Could you check a few things on this model? Use its own coordinates, in mm. Face numbers are marked on the shaded views. A direction names the side the tool comes from. Give positions to 0.01 mm unless a question says otherwise; leave off trailing zeros. Loops run counter-clockwise (first coordinate to the right, second up) from the corner with the lowest first, then second, coordinate; pieces in that order, holes last. Notation, with made-up numbers: (1.25, 71.5) - (33.25, 71.5) arc R16 ccw to (33.25, 81.5) - close; hole circle Ø10 at (24.5, -26.5). An arc over 180 degrees is marked (long way). Write each question's results on one line, items separated by ' | '. Start each with the question number.
(1) I need wall thicknesses on line 1 (X direction, y = -15, z = 22.25); line 2 (Y direction, x = 15, z = 22.2); line 3 (Y direction, x = -10, z = 13). Which ranges of each line are inside material? Lowest first, please.
(2) For pin 1 (1.8 mm diameter, centred on x = 15, y = -15, fed in from +Z); pin 2 (5 mm diameter, centred on x = -20, y = -15, fed in from +Z); pin 3 (10 mm diameter, centred on y = 21.5, z = 11.5, fed in from -X), each with a flat end and sliding along its axis, tell me the tip position at first contact or that it passes through.
(3) Suppose I cut it at C-C (z = 18.75). Please give me the cut outline in (x, y), and give its area (3 significant figures).
(4) Suppose I cut it at A-A (y = -15). Please give me the cut outline in (x, z).
(5) Suppose I cut it at B-B (x = 15). Please give me the cut outline in (y, z).
(6) Suppose I cut it at D-D (y = 2). Please give me the cut outline in (x, z).
(7) On a 3-axis mill with a long thin cutter (end or side, diameter ignored), from which of +Z, -Z, +X, -X, +Y, -Y can I reach the whole of each face in a straight line? I mean the marked faces 5, 6 and 7. Say none if no direction works.
(8) If we mould it in two halves opening along Y, with no side actions, what happens to the marked faces 1, 2, 3 and 4? For each: released by +Y, released by -Y, zero draft, split by the parting line, or undercut.
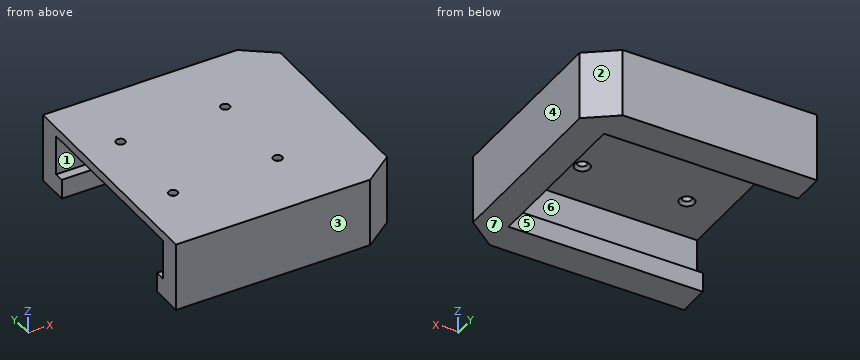
Autodesk Fusion 360 part; units mm, degrees
sketch "Sketch1" plane through (0, 0, 0) normal (0, 0, 1) x (1, 0, 0)
  line L0 (32.5, 30.5) -> (-32.5, 30.5)
  line L1 (-32.5, 30.5) -> (-32.5, -30.5)
  line L2 (-32.5, -30.5) -> (32.5, -30.5)
  line L3 (32.5, -30.5) -> (32.5, 30.5)
  line L4 (32.5, -27.25) -> (-32.5, -27.25)
  line L5 (-32.5, -27.25) -> (-32.5, 27.25)
  line L6 (-32.5, 27.25) -> (32.5, 27.25)
  line L7 (32.5, 27.25) -> (32.5, -27.25)
  line L8 (32.5, 38) -> (-32.5, 38)
  line L9 (42.5, -30.5) -> (42.5, 30.5)
  line L10 (32.5, 38) -> (42.5, 30.5)
  line L11 (-32.5, 38) -> (-32.5, 30.5)
  line L12 (1.75, 0) -> (22.5, 0)
  line L13 (-32.5, -38) -> (-32.5, -30.5)
  line L14 (32.5, -38) -> (-32.5, -38)
  line L15 (32.5, -38) -> (42.5, -30.5)
  line L16 (42.5, 30.5) -> (42.5, -30.5)
  dimension "d1" = 65
  dimension "d2" = 61
  dimension "d3" = 65
  dimension "d4" = 54.5
  dimension "d5" = 7.5
  dimension "d6" = 10
extrude "Extrude1" add sketch "Sketch1" along normal blind 6.6 contours L0 L1 L3 L6 | L0 L2 L3 L7 L8 L9 L10 L11 L13 L14 L15 L16 | L1 L2 L3 L4
extrude "Extrude2" add sketch "Sketch1" along normal blind 20 contours L0 L2 L3 L7 L8 L9 L10 L11 L13 L14 L15 L16
extrude "Extrude3" add sketch "Sketch1" along normal blind 23 and the other way blind -20
sketch "Sketch2" plane through (0, 0, 23) normal (0, 0, 1) x (-1, 0, 0)
  line L0 (-32.5, -38) -> (32.5, -38)
  line L1 (32.5, -38) -> (32.5, 38)
  line L2 (32.5, 38) -> (-32.5, 38)
  line L3 (-32.5, 38) -> (-42.5, 30.5)
  line L4 (-42.5, 30.5) -> (-42.5, -30.5)
  line L5 (-42.5, -30.5) -> (-32.5, -38)
  circle A0 centre (20, 15) radius 1.5
  circle A1 centre (-15, 15) radius 1.5
  line L6 (-1.75, 0) -> (-22.5, 0)
  circle A2 centre (20, -15) radius 1.5
  circle A3 centre (-15, -15) radius 1.5
  dimension "d15" = 3
  dimension "d16" = 3
extrude "Extrude4" cut sketch "Sketch2" against normal blind 5 contours A0 | A1 | A2 | A3
chamfer "Chamfer1" distance 1 angle 45 4 edges at (-18.6015, 15.5424, 20) (-18.6015, -14.4576, 20) (16.3985, -14.4576, 20) (16.3985, 15.5424, 20)
Output values:
1) line 1: -32.5 to -21.5, -18.5 to 13.5, 16.5 to 42.5 | line 2: -38 to -16.5, -13.5 to 13.5, 16.5 to 38 | line 3: -38 to -30.5, 30.5 to 38
2) pin 1: through | pin 2: z = 23 | pin 3: x = 32.5
3) outline: (-32.5, -38) - (32.5, -38) - (42.5, -30.5) - (42.5, 30.5) - (32.5, 38) - (-32.5, 38) - (-32.5, 30.5) - (32.5, 30.5) - (32.5, -30.5) - (-32.5, -30.5) - close | area: 1,660 mm2
4) outline: (-32.5, 20) - (-22.5, 20) - (-21.5, 21) - (-21.5, 23) - (-32.5, 23) - close; (-18.5, 21) - (-17.5, 20) - (12.5, 20) - (13.5, 21) - (13.5, 23) - (-18.5, 23) - close; (16.5, 21) - (17.5, 20) - (32.5, 20) - (32.5, 0) - (42.5, 0) - (42.5, 23) - (16.5, 23) - close
5) outline: (-38, 0) - (-27.25, 0) - (-27.25, 6.6) - (-30.5, 6.6) - (-30.5, 20) - (-17.5, 20) - (-16.5, 21) - (-16.5, 23) - (-38, 23) - close; (-13.5, 21) - (-12.5, 20) - (12.5, 20) - (13.5, 21) - (13.5, 23) - (-13.5, 23) - close; (16.5, 21) - (17.5, 20) - (30.5, 20) - (30.5, 6.6) - (27.25, 6.6) - (27.25, 0) - (38, 0) - (38, 23) - (16.5, 23) - close
6) outline: (-32.5, 20) - (32.5, 20) - (32.5, 0) - (42.5, 0) - (42.5, 23) - (-32.5, 23) - close
7) face 5: -Z, -X | face 6: -X | face 7: -Z, +X, -X, +Y, -Y
8) face 1: undercut | face 2: released by +Y | face 3: released by -Y | face 4: zero draft
